Here's how the part is built. I have some questions about the finished solid (model axes, mm). A direction names the side the tool comes from. Give positions to 0.01 mm unless a question says otherwise; leave off trailing zeros. Loops run counter-clockwise (first coordinate to the right, second up) from the corner with the lowest first, then second, coordinate; pieces in that order, holes last. Notation, with made-up numbers: (-36, 14) - (22, 14) arc R12 cw to (22, 28) - close; hole circle Ø2 at (-17, 44). An arc over 180 degrees is marked (long way). Use a Markdown table: item, result.
from build123d import *

# Parameters (mm, degrees)
SCHIZZO1_R                                           = 21.5
ESTRUSIONE_ESTRUSIONE1_DEPTH                         = 20
FORO_LAMATO_PER_VITE_M6_A_TESTA_CILINDRI_D           = 6.6
FORO_LAMATO_PER_VITE_M6_A_TESTA_CILINDRI_CBORE_D     = 11
FORO_LAMATO_PER_VITE_M6_A_TESTA_CILINDRI_CBORE_DEPTH = 6.4
CBORE_FOR_M6_HEX_SOCKET_HEAD_CAP_SCREW1_D            = 6.6
CBORE_FOR_M6_HEX_SOCKET_HEAD_CAP_SCREW1_DEPTH        = 50
CBORE_FOR_M6_HEX_SOCKET_HEAD_CAP_SCREW1_CBORE_D      = 11
CBORE_FOR_M6_HEX_SOCKET_HEAD_CAP_SCREW1_CBORE_DEPTH  = 6.4
CBORE_FOR_M6_HEX_SOCKET_HEAD_CAP_SCREW1_TIP          = 1.982840043
SCHIZZO7_W                                           = 15.52137419
SCHIZZO7_H                                           = 2
TAGLIO_ESTRUSIONE1_DEPTH                             = 136.882302012
CHAMFER1_SIZE                                        = 0.5
CHAMFER2_SIZE                                        = 0.5


with BuildPart() as part:
    # Schizzo1 → Estrusione-Estrusione1 (new body)
    with BuildSketch(Plane.XY):
        Polygon((0, 0), (108, 0), (108, 20), (88, 20), (88, 80), (20, 80), (20, 20), (0, 20), align=None)
        with Locations((54, 50)):
            Circle(SCHIZZO1_R, mode=Mode.SUBTRACT)
    extrude(amount=ESTRUSIONE_ESTRUSIONE1_DEPTH)

    # Foro lamato per Vite M6 a testa cilindrica-1 (through all)
    with Locations(Plane(origin=(9, 20, 10), x_dir=(0, 0, 1), z_dir=(0, 1, 0))):
        with Locations((0, 0), (0, 90)):
            CounterBoreHole(FORO_LAMATO_PER_VITE_M6_A_TESTA_CILINDRI_D / 2, FORO_LAMATO_PER_VITE_M6_A_TESTA_CILINDRI_CBORE_D / 2, FORO_LAMATO_PER_VITE_M6_A_TESTA_CILINDRI_CBORE_DEPTH)

    # CBORE for M6 Hex Socket Head Cap Screw1
    with Locations(Plane(origin=(26, 80, 10), x_dir=(0, 0, 1), z_dir=(0, 1, 0))):
        with Locations((0, 0)):
            CounterBoreHole(CBORE_FOR_M6_HEX_SOCKET_HEAD_CAP_SCREW1_D / 2, CBORE_FOR_M6_HEX_SOCKET_HEAD_CAP_SCREW1_CBORE_D / 2, CBORE_FOR_M6_HEX_SOCKET_HEAD_CAP_SCREW1_CBORE_DEPTH, depth=CBORE_FOR_M6_HEX_SOCKET_HEAD_CAP_SCREW1_DEPTH)
            with Locations((0, 0, -(CBORE_FOR_M6_HEX_SOCKET_HEAD_CAP_SCREW1_DEPTH + CBORE_FOR_M6_HEX_SOCKET_HEAD_CAP_SCREW1_TIP / 2))):  # 118° drill point
                Cone(0, CBORE_FOR_M6_HEX_SOCKET_HEAD_CAP_SCREW1_D / 2, CBORE_FOR_M6_HEX_SOCKET_HEAD_CAP_SCREW1_TIP, mode=Mode.SUBTRACT)

    # Schizzo7 → Taglio-Estrusione1 (cut, through all)
    with BuildSketch(Plane(origin=(0, 0, 0), x_dir=(-1, 0, 0), z_dir=(0, 0, -1))):
        with Locations((-27.66540179, 50)):
            Rectangle(SCHIZZO7_W, SCHIZZO7_H)
    extrude(amount=-TAGLIO_ESTRUSIONE1_DEPTH, mode=Mode.SUBTRACT)

    # Chamfer1
    chamfer1_edges = [part.edges().sort_by_distance(p)[0] for p in [
        (54.500135336, 71.494182112, 0),
    ]]
    chamfer(chamfer1_edges, length=CHAMFER1_SIZE)

    # Chamfer2
    chamfer2_edges = [part.edges().sort_by_distance(p)[0] for p in [
        (54.500135336, 28.505817888, 20),
    ]]
    chamfer(chamfer2_edges, length=CHAMFER2_SIZE)


solid = part.part
(1) Will these pins go through, and if not, where does the flat tip stop? pin 1 (12 mm diameter, centred on x = 9.5, z = 10.5, fed in from +Y); pin 2 (5.5 mm diameter, centred on x = 26, z = 10, fed in from -Y); pin 3 (6 mm diameter, centred on y = 65, z = 12, fed in from -X); pin 4 (10 mm diameter, centred on y = 28, z = 12, fed in from +X).
A:
| item | result |
|---|---|
| pin 1 | y = 20 |
| pin 2 | y = 0 |
| pin 3 | x = 20 |
| pin 4 | x = 88 |
(2) If I drill on line 1 (X direction, y = 17, z = 10); line 2 (X direction, y = 5.5, z = 10); line 3 (Y direction, x = 55, z = 16), over which ranges is the centre line in solid material (lowest first)?
A:
| item | result |
|---|---|
| line 1 | 0 to 3.5, 14.5 to 93.5, 104.5 to 108 |
| line 2 | 0 to 5.7, 12.3 to 95.7, 102.3 to 108 |
| line 3 | 0 to 28.52, 71.48 to 80 |
(3) On a 3-axis mill with a long thin cutter (end or side, diameter ignored), from which of +Z, -Z, +X, -X, +Y, -Y can I reach the whole of each face in a straight line? I mean faces 4 (the face through (20, 35, 10)), 5 (the face through (88, 50, 10)), 6 (the face through (108, 10, 10)), 7 (the face through (29, 49, 8)), 8 (the face through (23.992, 62.142, 12.619)). Say none if no direction works.
A:
| item | result |
|---|---|
| face 4 | +Z, -Z, -X, +Y |
| face 5 | +Z, -Z, +X, +Y |
| face 6 | +Z, -Z, +X, +Y, -Y |
| face 7 | +Z, -Z, -X |
| face 8 | +Y |
(4) We'd pull the mould along X, two halves only. Please class faces 1 (the face through (15, 20, 10)), 2 (the face through (6.992, 6.705, 12.619)), 3 (the face through (0, 10, 10)): pulls with the +X half, pulls with the -X half, needs draft (parallel to the pull), parting line crosses it, or undercut.
A:
| item | result |
|---|---|
| face 1 | needs draft |
| face 2 | undercut |
| face 3 | pulls with the -X half |
(5) Suppose I cut it at B-B on z = 2.25. Write out the boundary of the cut face in (x, y), plus the area to 3 significant figures.
A:
| item | result |
|---|---|
| outline | (0, 0) - (108, 0) - (108, 20) - (88, 20) - (88, 80) - (20, 80) - (20, 51) - (32.52, 51) arc R21.5 cw (long way) to (32.52, 49) - (20, 49) - (20, 20) - (0, 20) - close |
| area | 4,760 mm2 |
(6) Suppose I cut it at C-C on x = 54. Write out the boundary of the cut face in (y, z), plus the area to 4 significant figures.
A:
| item | result |
|---|---|
| outline | (0, 0) - (28, 0) - (28.5, 0.5) - (28.5, 19.5) - (28, 20) - (0, 20) - close; (71.5, 0.5) - (72, 0) - (80, 0) - (80, 20) - (72, 20) - (71.5, 19.5) - close |
| area | 739.5 mm2 |
(7) Suppose I cut it at A-A on x = 99. Write out the boundary of the cut face in (y, z), plus the area to 3 significant figures.
A:
| item | result |
|---|---|
| outline | (0, 0) - (20, 0) - (20, 4.5) - (13.6, 4.5) - (13.6, 6.7) - (0, 6.7) - close; (0, 13.3) - (13.6, 13.3) - (13.6, 15.5) - (20, 15.5) - (20, 20) - (0, 20) - close |
| area | 240 mm2 |
(8) Suppose I cut it at D-D on y = 64. Count the separate pieces of the cut face and the enclosed holes in it, plus the area to 3 significant figures.
A:
| item | result |
|---|---|
| separate pieces | 2 |
| enclosed holes | 1 |
| area | 672 mm2 |
